Part model, mm, in its own coordinate system. A direction names the side the tool comes from. Round coordinates to 2 decimals unless told otherwise and drop trailing zeros. Order: outer loops, then holes, each group sorted by start corner. A loop starts at its lowest first (then second) coordinate and runs counter-clockwise, first axis right, second up. Notation, with made-up numbers: (13.25, 64.25) - (68.25, 64.25) arc R32 ccw to (68.25, 93.25) - close; hole circle Ø3 at (34.5, -3.75). An arc over 180 degrees is marked (long way). Return JSON: item names as keys, results as strings. Group by question number.
Item 1: Saw through at A-A on x = 0. List the corners of the cut face in (y, z).
Item 2: Saw through at C-C on x = 10. List the corners of the cut face in (y, z), and give its area (3 significant figures).
Item 3: Tool access for faces 1 (the face through (-5.961, 26.846, 102.686)), 2 (the face through (-14.4, -18.2, 101.7)): list every direction of +Z, -Z, +X, -X, +Y, -Y with a clear straight run to the whole face (end or side of a thin tool).
Item 4: Two-plate mould, pull along Y, no slides. Class faces 3 (the face through (-2.994, -22.804, 95.261)), 4 (the face through (-0.3, 5.3, 101.7)), 5 (the face through (0, -6, 103.7)), 6 (the face through (19.961, -10.382, 95.261)): released by +Y, released by -Y, zero draft, split by the parting line, or undercut.
Item 5: Drop flat-ended pins along their axis: pin 1 (5 mm diameter, centred on x = 19, z = 93.5, fed in from -Y); pin 2 (2 mm diameter, centred on x = -13, z = 95, fed in from +Y); pin 3 (13.5 mm diameter, centred on x = -3.5, y = -2.5, fed in from -Z). Give the stop position or say it passes through.
Item 6: Saw through at D-D on y = 24.5. List the corners of the cut face in (x, z).
Item 7: Probe probe 1 along Y at (x, z) = (0, 102.9); probe 2 along Y at (x, z) = (0, 98.75). List the from-to ranges inside material, lowest first.
Autodesk Inventor part; units mm, degrees
ref_plane "Work Plane2" through (0, 0, 89) normal (0, 0, 1) x (1, 0, 0)
ref_plane "YZ Plane" through (0, 0, 0) normal (1, 0, 0) x (0, 1, 0)
ref_plane "XZ Plane" through (0, 0, 0) normal (0, 1, 0) x (-1, 0, 0)
ref_plane "Work Plane1" through (0, 0, 76.3) normal (0, 0, 1) x (1, 0, 0)
ref_plane "Work Plane2" through (0, 0, 89) normal (0, 0, 1) x (1, 0, 0)
sketch "Sketch4" plane through (0, 0, 89) normal (0, 0, 1) x (1, 0, 0)
  circle A0 centre (0, 0) radius 23.5
  circle A1 centre (0, 0) radius 23
  dimension "d20" = 46
extrude "Extrusion4" add sketch "Sketch4" along normal blind 12.7 contours A1
sketch "Sketch5" plane through (0, 0, 101.7) normal (0, 0, 1) x (1, 0, 0)
  circle A0 centre (0, 0) radius 23
  circle A1 centre (0, 0) radius 23
hole "Hole2" at (0, 0, 101.7) direction (0, 0, -1) diameter 45 depth 12.8
sketch "Sketch6" plane through (0, 0, 101.7) normal (0, 0, 1) x (1, 0, 0)
  circle A0 centre (0, 0) radius 22.5
  circle A1 centre (0, 0) radius 23
  line L0 (0, -38.5) -> (0, 38.5)
  line L1 (-38.5, 0) -> (38.5, 0)
  circle A2 centre (0, 0) radius 27.5
  dimension "d30" = 55
extrude "Extrusion5" add sketch "Sketch6" along normal blind 2
sketch "Sketch7" plane through (0, 0, 103.7) normal (0, 0, 1) x (1, 0, 0)
  circle A0 centre (0, 0) radius 27.5
  line L0 (0, -38.5) -> (0, 38.5)
  line L1 (-38.5, 0) -> (38.5, 0)
hole "Hole3" at (0, 0, 103.7) direction (0, 0, -1) diameter 10 depth 8 tip angle 118
properties part number "Plastic Lid"
Filled in:
{
 "1": {"outline": "(-27.5, 101.7) - (-23, 101.7) - (-23, 89) - (-22.5, 89) - (-22.5, 101.7) - (-5, 101.7) - (-5, 103.7) - (-27.5, 103.7) - close; (5, 101.7) - (22.5, 101.7) - (22.5, 89) - (23, 89) - (23, 101.7) - (27.5, 101.7) - (27.5, 103.7) - (5, 103.7) - close"},
 "2": {"outline": "(-25.62, 101.7) - (-20.71, 101.7) - (-20.71, 89) - (-20.16, 89) - (-20.16, 101.7) - (20.16, 101.7) - (20.16, 89) - (20.71, 89) - (20.71, 101.7) - (25.62, 101.7) - (25.62, 103.7) - (-25.62, 103.7) - close", "area": "117 mm^2"},
 "3": {"face 1": "+Z, -Z", "face 2": "-Z"},
 "4": {"face 3": "split by the parting line", "face 4": "undercut", "face 5": "zero draft", "face 6": "undercut"},
 "5": {"pin 1": "stops at y = -16.02", "pin 2": "stops at y = 19.62", "pin 3": "stops at z = 101.7"},
 "6": {"outline": "(-12.49, 101.7) - (12.49, 101.7) - (12.49, 103.7) - (-12.49, 103.7) - close"},
 "7": {"probe 1": "y = -27.5 to -5, 5 to 27.5", "probe 2": "y = -23 to -22.5, 22.5 to 23"}
}
